Model file for the job. Use its own axes, mm. Round coordinates to 2 decimals unless told otherwise and drop trailing zeros. Loops run counter-clockwise (first coordinate to the right, second up) from the corner with the lowest first, then second, coordinate; pieces in that order, holes last. Notation, with made-up numbers: (63, 77) -> (86, 77) arc R20 ccw to (86, 94) -> close; hole circle Ø11 at (24.25, 43.5). An arc over 180 degrees is marked (long way). Use a Markdown table: item, result. Add a question column.
```python
from build123d import *

# Parameters (mm, degrees)
BOSS_EXTRUDE1_DEPTH = 2
CUT_EXTRUDE1_DEPTH  = 1
SCALE1_SCALE        = 0.5


with BuildPart() as part:
    # Sketch1 → Boss-Extrude1 (new body)
    with BuildSketch(Plane.XY):
        Polygon((-48.310810811, 14.243974201), (151.689189189, 14.243974201), (151.689189189, 4.243974201), (126.689189189, 4.243974201), (126.689189189, -30.756025799), (151.689189189, -30.756025799), (151.689189189, -40.756025799), (-48.310810811, -40.756025799), (-48.310810811, -30.756025799), (-23.310810811, -30.756025799), (-23.310810811, 4.243974201), (-48.310810811, 4.243974201), align=None)
    extrude(amount=BOSS_EXTRUDE1_DEPTH)

    # Sketch3 → Cut-Extrude1 (cut)
    with BuildSketch(Plane.XY.offset(2)):
        with BuildLine():
            add(Edge.make_bspline(
                [(37.189484824, -10.718294686), (33.474166953, -10.624199422), (35.300627772, -23.216467907), (74.220048032, -9.046257892), (87.664897587, -2.594986042), (98.853365994, 3.337442933)],
                knots=[0, 0, 0, 0, 0.51776511, 0.592619661, 1, 1, 1, 1], degree=3))
            add(Edge.make_bspline(
                [(37.189484824, -10.718294686), (30.815944463, -10.332745105), (29.156875012, -24.169852988), (43.250186434, -25.85327449), (65.190161886, -16.178918043), (83.996504619, -6.384768657), (98.853365994, 3.337442933)],
                knots=[0, 0, 0, 0, 0.163170519, 0.29176393, 0.388322168, 1, 1, 1, 1], degree=3))
        make_face()
    extrude(amount=-CUT_EXTRUDE1_DEPTH, mode=Mode.SUBTRACT)


with BuildPart() as part_1:
    # Scale1: scaled about (51.685288163, -13.204114524, 0.992436244)
    add(part.part.scale(SCALE1_SCALE).moved(Location((25.842644082, -6.602057262, 0.496218122))))


solid = part_1.part
```
1) Pull direction Y, two halves, no side cores. Call faces 1 (the face through (52, -13, 0.496)), 2 (the face through (51.5, -15.4, 0.996)): +Y half, -Y half, draft (parallel to the pull), parting line (faces both ways), or undercut.
2) Wall check: probe 1 along X at (y, z) = (-20.5, 1.35); probe 2 along X at (y, z) = (-11, 1.2); probe 3 along Y at (x, z) = (43, 1.2). Give the ranges that are in metal, low to high. Write a range as from..to.
3) Pin check, flat tip, straight feed: pin 1 Ø0.5 at (y, z) = (-17.5, 1) entering from -X. Stop position of the tip, or through.
4) Cut at A-A on z = 0.65. Write the cut outline in (x, y).
Established:
| question | item | result |
|---|---|---|
| 1 | face 1 | draft |
| 1 | face 2 | undercut |
| 2 | probe 1 | x = 14.19..89.19 |
| 2 | probe 2 | x = 14.19..62.63, 65.1..89.19 |
| 2 | probe 3 | y = -26.98..-18.26, -12.21..0.52 |
| 3 | pin 1 | stops at x = 14.19 |
| 4 | outline | (1.69, -26.98) -> (101.69, -26.98) -> (101.69, -21.98) -> (89.19, -21.98) -> (89.19, -4.48) -> (101.69, -4.48) -> (101.69, 0.52) -> (1.69, 0.52) -> (1.69, -4.48) -> (14.19, -4.48) -> (14.19, -21.98) -> (1.69, -21.98) -> close |
